For this review, take the finished solid that the model builds, in its own axes (mm). Face numbers are marked on the shaded views. A direction names the side the tool comes from. Round coordinates to 2 decimals unless told otherwise and drop trailing zeros. Order: outer loops, then holes, each group sorted by start corner. A loop starts at its lowest first (then second) coordinate and runs counter-clockwise, first axis right, second up. Notation, with made-up numbers: (-23, 82) - (33, 82) arc R23 ccw to (33, 102) - close; hole circle Ø7 at (47, 36). An arc over 180 degrees is marked (long way). One line per item, written item: value.
```python
from build123d import *

# Parameters (mm, degrees)
BASPROSKE_W             = 5
BASPROSKE_H             = 4.2
TOOTHCUT_DEPTH          = 8.764019578
TEETHCUTS_COUNT         = 10
TEETHCUTS_ANGLE         = 324
BORSKE_R                = 1.5
BORE_DEPTH              = 50.0000508
CROQUIS1_R              = 4.25
CROQUIS1_R_2            = 3.25
SALIENTE_EXTRUIR1_DEPTH = 5
CROQUIS2_R              = 3.25
SALIENTE_EXTRUIR2_DEPTH = 2
SALIENTE_EXTRUIR3_DEPTH = 2


with BuildPart() as part:
    # BasProSke → Base-Revolve (revolve)
    with BuildSketch(Plane(origin=(0, 0, 0), x_dir=(1, 0, 0), z_dir=(0, 1, 0)), mode=Mode.PRIVATE) as base_revolve_sk:
        with Locations((2.5, 2.1)):
            Rectangle(BASPROSKE_W, BASPROSKE_H)
    revolve(base_revolve_sk.sketch.rotate(Axis((-10, 0, 0), (1, 0, 0)), 180), axis=Axis((-10, 0, 0), (1, 0, 0)))

    # TooCutSke → ToothCut (cut, through all)
    with BuildSketch(Plane(origin=(0, 0, 0), x_dir=(0, 0, -1), z_dir=(1, 0, 0))):
        with BuildLine():
            ThreePointArc((0.415506654, 2.590893711), (0, 2.624), (-0.415506654, 2.590893711))
            ThreePointArc((-0.415506654, 2.590893711), (-0.596160737, 3.451685568), (-1.254578949, 4.034852763))
            ThreePointArc((-1.254578949, 4.034852763), (0, 4.2254), (1.254578949, 4.034852763))
            ThreePointArc((1.254578949, 4.034852763), (0.596160737, 3.451685568), (0.415506654, 2.590893711))
        make_face()
    toothcut = extrude(amount=TOOTHCUT_DEPTH, mode=Mode.SUBTRACT)

    # TeethCuts: ToothCut ×10 about axis
    teethcuts_axis = Axis((-10, 0, 0), (1, 0, 0))
    for i in range(1, TEETHCUTS_COUNT):
        add(toothcut.rotate(teethcuts_axis, i * TEETHCUTS_ANGLE / (TEETHCUTS_COUNT - 1)), mode=Mode.SUBTRACT)

    # BorSke → Bore (cut, symmetric)
    with BuildSketch(Plane(origin=(0, 0, 0), x_dir=(0, 0, -1), z_dir=(1, 0, 0))):
        with Locations(Location((0, 0, 0), (0, 0, 180))):
            Circle(BORSKE_R)
    extrude(amount=BORE_DEPTH, both=True, mode=Mode.SUBTRACT)

    # Croquis1 → Saliente-Extruir1 (add)
    with BuildSketch(Plane.ZY):
        Circle(CROQUIS1_R)
        with Locations(Location((0, 0, 0), (0, 0, 189.396976621))):
            Circle(CROQUIS1_R_2, mode=Mode.SUBTRACT)
    extrude(amount=SALIENTE_EXTRUIR1_DEPTH)

    # Croquis2 → Saliente-Extruir2 (add)
    with BuildSketch(Plane.ZY):
        Circle(CROQUIS2_R)
    extrude(amount=SALIENTE_EXTRUIR2_DEPTH)

    # Croquis3 → Saliente-Extruir3 (add)
    with BuildSketch(Plane.ZY.offset(2)):
        with BuildLine():
            Line((-1.5, 2.883140649), (-1.5, -2.883140649))
            ThreePointArc((-1.5, -2.883140649), (-3.25, 0), (-1.5, 2.883140649))
        make_face()
    extrude(amount=SALIENTE_EXTRUIR3_DEPTH)


solid = part.part
```
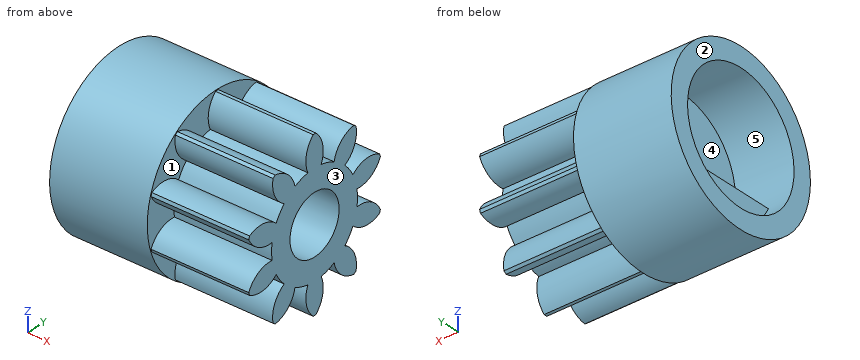
Item 1: Take a section at C-C (x = -1.5). Write out the cut boundary in (y, z).
Returned:
outline: circle Ø8.5 at (0, 0)
Item 2: Machinability: for the marked faces 1 and 2, which of the approach directions +Z, -Z, +X, -X, +Y, -Y give a long, thin tool a straight path to every point of the face, cutting with its end or side? Answer none if there is none.
Returned:
face 1: +X
face 2: +Z, -Z, -X, +Y, -Y
Item 3: Take a section at A-A (z = 0). Write out the cut boundary in (x, y).
Returned:
outline: (-5, -4.25) - (0, -4.25) - (0, -2.62) - (5, -2.62) - (5, -1.5) - (0, -1.5) - (0, 1.5) - (5, 1.5) - (5, 2.62) - (0, 2.62) - (0, 4.25) - (-5, 4.25) - (-5, 3.25) - (-2, 3.25) - (-2, -3.25) - (-5, -3.25) - close
Item 4: Take a section at D-D (z = 1). Write out the cut boundary in (x, y), plus the area to 3 significant figures.
Returned:
outline: (-5, -4.13) - (0, -4.13) - (0, -3.89) - (5, -3.89) - (5, -1.12) - (0, -1.12) - (0, 1.12) - (5, 1.12) - (5, 3.89) - (0, 3.89) - (0, 4.13) - (-5, 4.13) - (-5, 3.09) - (-2, 3.09) - (-2, -3.09) - (-5, -3.09) - close
area: 50.5 mm^2
Item 5: For P1, Ø4, axis at y = -0.5, z = 0, coming from the -X side; P2, Ø1, axis at x = -2.5, y = 1, coming from the +Z side; P3, Ø4, axis at y = 0, z = 0, coming from the +X side; P4, Ø1.5, axis at y = 0.5, z = 0.5, coming from the +X side, all flat-tipped, find the tip position at first contact; note any pin that passes through.
Returned:
P1: x = -4
P2: z = 4.22
P3: x = 5
P4: x = 0
Item 6: Wall thickness on line 1 (Y direction, x = 3.5, z = 0); line 2 (Y direction, x = -2.8, z = 0); line 3 (X direction, y = 2.25, z = -2.25): over which ranges is each line inside the solid? List them lowest first.
Returned:
line 1: -2.62 to -1.5, 1.5 to 2.62
line 2: -4.25 to -3.25, 3.25 to 4.25
line 3: -4 to 5
Item 7: Take a section at B-B (y = -3.5). Write out the cut boundary in (x, z).
Returned:
outline: (-5, -2.41) - (0, -2.41) - (0, -1.54) - (5, -1.54) - (5, -0.63) - (0, -0.63) - (0, 0.63) - (5, 0.63) - (5, 1.54) - (0, 1.54) - (0, 2.41) - (-5, 2.41) - close
Item 8: The part is to be moulded in two halves that separate along X. For the marked faces 3, 4 and 5, say which applies: +X half, -X half, draft (parallel to the pull), parting line (faces both ways), or undercut.
Returned:
face 3: +X half
face 4: -X half
face 5: draft
